from build123d import *

# Parameters (mm, degrees)
F0_W     = 116.467763
F0_H     = 90.848792
F1_DEPTH = 127
F2_R     = 31.135963
F3_DEPTH = 127
F4_R     = 5.08


with BuildPart() as f1:
    # F0 (on Top) → F1 (new body)
    with BuildSketch(Plane.XY):
        with Locations((2.364828, -2.561895)):
            Rectangle(F0_W, F0_H)
    extrude(amount=F1_DEPTH)

    # F2 (on face) → F3 (cut)
    with BuildSketch(Plane.XY.offset(127)):
        Circle(F2_R)
    extrude(amount=-F3_DEPTH, mode=Mode.SUBTRACT)

    # F4
    f4_edges = [f1.edges().sort_by_distance(p)[0] for p in [
        (2.364827, 42.862501, 127),
        (-55.869054, -2.561895, 127),
        (2.364827, -47.986291, 127),
        (60.598709, -2.561895, 127),
        (-31.135963, 0, 127),
        (-55.869054, 42.862501, 63.5),
        (-55.869054, -2.561895, 0),
        (-55.869054, -47.986291, 63.5),
        (2.364827, 42.862501, 0),
        (60.598709, 42.862501, 63.5),
        (31.135963, 0, 63.5),
        (-31.135963, 0, 0),
        (60.598709, -2.561895, 0),
        (2.364827, -47.986291, 0),
        (60.598709, -47.986291, 63.5),
    ]]
    fillet(f4_edges, radius=F4_R)


solid = f1.part
Design review of the part built by this model. Coordinates are the model's own, in mm. Coordinates: 2 decimals unless noted, no trailing zeros. Order: outer loops, then holes, each group sorted by start corner. A loop starts at its lowest first (then second) coordinate and runs counter-clockwise, first axis right, second up.
Item 1: Take a section at B-B, the plane y = 0. Write out the cut boundary in (x, z).
Item 2: Take a section at A-A, the plane x = 0. Write out the cut boundary in (y, z), then the cut area to 3 significant figures.
Item 3: For pin 1 Ø6 at (x, y) = (12, 23) entering from +Z, flat-tipped, find the tip position at first contact; note if it passes through.
Item 4: The part is to be moulded in two halves that separate along Y. For faces 1 (the cylindrical face through (59.07, -2, 1.45)), 2 (the cylindrical face through (59.071, 41.414, 64.318)), 3 (the cylindrical face through (29.7, 9.35, 64.32)), 4 (the cylindrical face through (-54.42, -46.46, 64.32)), say which applies: pulls with the +Y half, pulls with the -Y half, needs draft (parallel to the pull), parting line crosses it, or undercut.
Item 5: Take a section at C-C, the plane z = 17.5. Write out the cut boundary in (x, y), then the cut area to 3 significant figures.
Item 6: For line 1 (Y direction, x = 0, z = 87.5); line 2 (Z direction, x = 9.5, y = 38); line 3 (X direction, y = 22.5, z = 22.5), list the stretches that pass through material, from the lowest coordinate up.
The answers:
1. outline: (-55.87, 5.08) arc R5.08 ccw to (-50.79, 0) - (-36.22, 0) arc R5.08 ccw to (-31.14, 5.08) - (-31.14, 121.92) arc R5.08 ccw to (-36.22, 127) - (-50.79, 127) arc R5.08 ccw to (-55.87, 121.92) - close; (31.14, 5.08) arc R5.08 ccw to (36.22, 0) - (55.52, 0) arc R5.08 ccw to (60.6, 5.08) - (60.6, 121.92) arc R5.08 ccw to (55.52, 127) - (36.22, 127) arc R5.08 ccw to (31.14, 121.92) - close
2. outline: (-47.99, 5.08) arc R5.08 ccw to (-42.91, 0) - (-36.22, 0) arc R5.08 ccw to (-31.14, 5.08) - (-31.14, 121.92) arc R5.08 ccw to (-36.22, 127) - (-42.91, 127) arc R5.08 ccw to (-47.99, 121.92) - close; (31.14, 5.08) arc R5.08 ccw to (36.22, 0) - (37.78, 0) arc R5.08 ccw to (42.86, 5.08) - (42.86, 121.92) arc R5.08 ccw to (37.78, 127) - (36.22, 127) arc R5.08 ccw to (31.14, 121.92) - close
2. area: 3,580 mm2
3. pin 1: passes through
4. face 1: needs draft
4. face 2: pulls with the +Y half
4. face 3: undercut
4. face 4: pulls with the -Y half
5. outline: (-55.87, -42.91) arc R5.08 ccw to (-50.79, -47.99) - (55.52, -47.99) arc R5.08 ccw to (60.6, -42.91) - (60.6, 37.78) arc R5.08 ccw to (55.52, 42.86) - (-50.79, 42.86) arc R5.08 ccw to (-55.87, 37.78) - close; hole circle Ø62.27 at (0, 0)
5. area: 7,510 mm2
6. line 1: y = -47.99 to -31.14, 31.14 to 42.86
6. line 2: z = 0 to 127
6. line 3: x = -55.87 to -21.52, 21.52 to 60.6
